Could you check a few things on this drawing? It's one solid part, dimensions in mm from its lowest x, y, z. Give positions to 0.01 mm unless a question says otherwise; leave off trailing zeros. Loops run counter-clockwise (first coordinate to the right, second up) from the corner with the lowest first, then second, coordinate; pieces in that order, holes last.
Q1. Suppose I cut it at A-A (z = 0.5). List the corners of the cut face in (x, y) for me (1 decimal), and give its area (3 significant figures).
Q2. I need wall thicknesses on probe 1 along X at (y, z) = (37, 0.95) (1 decimal); probe 2 along X at (y, z) = (35.5, 2.55) (1 decimal); probe 3 along Y at (x, z) = (89, 0.3). Which ranges of each line are inside material? Lowest first, please.
Q3. Suppose I cut it at D-D (y = 41). List the corners of the cut face in (x, z) for me (1 decimal).
Q4. Suppose I cut it at B-B (y = 17). Count the separate pieces of the cut face and the enclosed holes in it.
Q5. Suppose I cut it at C-C (x = 89). List the corners of the cut face in (y, z) for me (1 decimal).
Q6. I'm going to push a flat-ended pin straight in: P1, Ø10, axis at x = 48.5, y = 18, coming from the -Z side. Where does the tip first touch, or does it pass through?
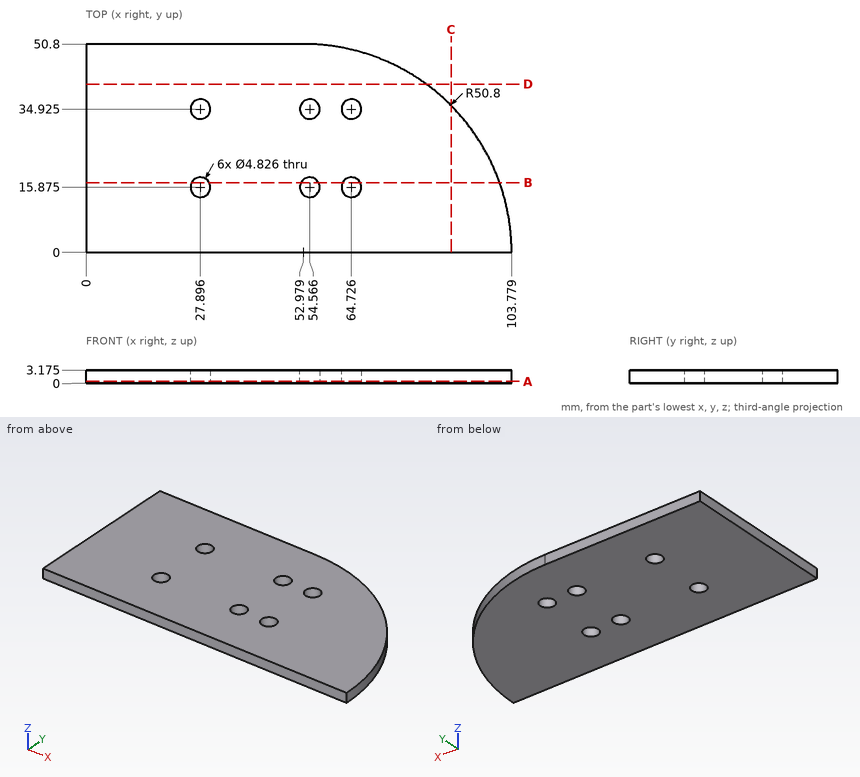
Solutions:
1. outline: (0, 0) - (103.8, 0) arc R50.8 ccw to (53, 50.8) - (0, 50.8) - close; hole circle Ø4.8 at (27.9, 15.9); hole circle Ø4.8 at (27.9, 34.9); hole circle Ø4.8 at (54.6, 15.9); hole circle Ø4.8 at (54.6, 34.9); hole circle Ø4.8 at (64.7, 15.9); hole circle Ø4.8 at (64.7, 34.9)
1. area: 4,610 mm2
2. probe 1: x = 0 to 26.7, 29.1 to 53.3, 55.8 to 63.5, 66 to 87.8
2. probe 2: x = 0 to 25.6, 30.2 to 52.2, 56.9 to 62.4, 67.1 to 89.3
2. probe 3: y = 0 to 35.82
3. outline: (0, 0) - (83, 0) - (83, 3.2) - (0, 3.2) - close
4. separate pieces: 4
4. enclosed holes: 0
5. outline: (0, 0) - (35.8, 0) - (35.8, 3.2) - (0, 3.2) - close
6. P1: stops at z = 0
